```python
from build123d import *

# Parameters (mm, degrees)
BOSS_EXTRUDE3_DEPTH = 4.5
CIRPATTERN1_COUNT   = 12
CIRPATTERN2_COUNT   = 6
SKETCH11_R          = 6.35
CUT_EXTRUDE1_DEPTH  = 10


with BuildPart() as part:
    # Sketch5 → Boss-Extrude3 (new body)
    with BuildSketch(Plane(origin=(0, 0, 0), x_dir=(1, 0, 0), z_dir=(0, 1, 0))):
        with BuildLine():
            ThreePointArc((-45.876558414, 184.378256278), (0.010243817, -189.999999724), (45.856676704, 184.383202059))
            ThreePointArc((45.856676704, 184.383202059), (37.985823171, 188.339968607), (32.578557994, 195.294666309))
            ThreePointArc((32.578557994, 195.294666309), (-0.011645544, 215.998911827), (-32.599616361, 195.291152239))
            ThreePointArc((-32.599616361, 195.291152239), (-38.006131584, 188.335871514), (-45.876558414, 184.378256278))
        make_face()
        with BuildLine():
            Line((-47.367120943, -99.136010081), (-47.045154091, -81.484597135))
            Line((-47.045154091, -81.484597135), (-62.170742689, -90.589135081))
            ThreePointArc((-62.170742689, -90.589135081), (-127.630493883, -73.6875), (-109.537863632, -8.546875))
            Line((-109.537863632, -8.546875), (-94.090308181, 0))
            Line((-94.090308181, 0), (-109.537863632, 8.546875))
            ThreePointArc((-109.537863632, 8.546875), (-127.630493883, 73.6875), (-62.170742689, 90.589135081))
            Line((-62.170742689, 90.589135081), (-47.045154091, 81.484597135))
            Line((-47.045154091, 81.484597135), (-47.367120943, 99.136010081))
            ThreePointArc((-47.367120943, 99.136010081), (0, 147.375), (47.367120943, 99.136010081))
            Line((47.367120943, 99.136010081), (47.045154091, 81.484597135))
            Line((47.045154091, 81.484597135), (62.170742689, 90.589135081))
            ThreePointArc((62.170742689, 90.589135081), (127.630493883, 73.6875), (109.537863632, 8.546875))
            Line((109.537863632, 8.546875), (94.090308181, 0))
            Line((94.090308181, 0), (109.537863632, -8.546875))
            ThreePointArc((109.537863632, -8.546875), (127.630493883, -73.6875), (62.170742689, -90.589135081))
            Line((62.170742689, -90.589135081), (47.045154091, -81.484597135))
            Line((47.045154091, -81.484597135), (47.367120943, -99.136010081))
            ThreePointArc((47.367120943, -99.136010081), (0, -147.375), (-47.367120943, -99.136010081))
        make_face(mode=Mode.SUBTRACT)
    extrude(amount=-BOSS_EXTRUDE3_DEPTH)

    # Sketch7 → CSK for M5 Flat Head Machine Screw1 (revolve, cut)
    with BuildSketch(Plane(origin=(-170, 0, 0), x_dir=(0, 0, 1), z_dir=(1, 0, 0))):
        Polygon((0, 0), (0, 4.5), (2.75, 4.5), (2.75, 2.45), (5.2, 0), align=None)
    csk_for_m5_flat_head_machine_screw1 = revolve(axis=Axis((-170, 6.35, 0), (0, -1, 0)), mode=Mode.SUBTRACT)

    # CirPattern1: CSK for M5 Flat Head Machine Screw1 ×12 about axis, 1 skipped
    cirpattern1_axis = Axis((0, 0, 0), (0, 1, 0))
    add([csk_for_m5_flat_head_machine_screw1.rotate(cirpattern1_axis, i * 360 / CIRPATTERN1_COUNT) for i in range(1, CIRPATTERN1_COUNT) if i not in (9,)], mode=Mode.SUBTRACT)

    # Sketch9 → CSK for M5 Flat Head Machine Screw2 (revolve, cut)
    with BuildSketch(Plane(origin=(-140, 0, 0), x_dir=(0, 0, 1), z_dir=(1, 0, 0))):
        Polygon((0, 0), (0, 4.5), (2.75, 4.5), (2.75, 2.45), (5.2, 0), align=None)
    csk_for_m5_flat_head_machine_screw2 = revolve(axis=Axis((-140, 6.35, 0), (0, -1, 0)), mode=Mode.SUBTRACT)

    # CirPattern2: CSK for M5 Flat Head Machine Screw2 ×6 about axis
    cirpattern2_axis = Axis((0, 0, 0), (0, 1, 0))
    for i in range(1, CIRPATTERN2_COUNT):
        add(csk_for_m5_flat_head_machine_screw2.rotate(cirpattern2_axis, i * 360 / CIRPATTERN2_COUNT), mode=Mode.SUBTRACT)

    # Sketch11 → Cut-Extrude1 (cut)
    with BuildSketch(Plane(origin=(0, 0, 0), x_dir=(1, 0, 0), z_dir=(0, 1, 0))):
        with Locations((-0.009704669, 179.999999411)):
            Circle(SKETCH11_R)
    extrude(amount=-CUT_EXTRUDE1_DEPTH, mode=Mode.SUBTRACT)


solid = part.part
```
Can you work these out from the model? Positions are in its coordinate system, mm. A direction names the side the tool comes from. Coordinates: 2 decimals unless noted, no trailing zeros. Loops run counter-clockwise (first coordinate to the right, second up) from the corner with the lowest first, then second, coordinate; pieces in that order, holes last. Notation, with made-up numbers: M -11.5,-27 L 36.5,-27 A23 ccw 36.5,10 Z; hole C 64.25,-24 d4. An arc over 180 degrees is marked long. Put each result on its own line as item: value. Start each with the question number.
(1) Which directions (+Z, -Z, +X, -X, +Y, -Y) give clear straight access to the entire face, cutting with the end or side of a thin tool? Please do faces 4 (the face through (-147.85, -2.3, -87.83)), 5 (the face through (54.71, -2.22, 86.1)).
(2) Imagine slicing it at A-A on z = -136. List the corners of the cut face in (x, y) for me, and give its area (3 significant figures).
(3) I need wall thicknesses on probe 1 along X at (y, z) = (-2.95, 0); probe 2 along Z at (x, y) = (127.5, -1.15); probe 3 along X at (y, z) = (-1.15, 1). Which ranges of each line are inside material? Lowest first, please.
(4) Will these pins go through, and if not, where does the flat tip stop? pin 1 Ø3.5 at (x, z) = (-147.22, -85) entering from +Y; pin 2 Ø2 at (y, z) = (-0.5, -133) entering from -X; pin 3 Ø6.5 at (x, z) = (-70, 121.24) entering from +Y; pin 4 Ø7 at (x, z) = (-70, -121.24) entering from +Y.
(5) Imagine slicing it at C-C on x = 102.5. List the corners of the cut face in (y, z) for me, and give its area (3 significant figures).
(6) We'd pull the mould along X, two halves only. Please class faces 1 (the face through (69.87, -2.3, -124.14)), 2 (the face through (0.559, -2.218, -215.994)), 3 (the face through (-45, 0, 119)): +X half, -X half, draft (parallel to the pull), parting line (faces both ways), or undercut.
(7) Imagine slicing it at B-B on x = -39. List the corners of the cut face in (y, z) for me, and give its area (3 significant figures).
Worked answers:
1. face 4: +Y
1. face 5: +Y, -Y
2. outline: M -132.68,-4.5 L -30.8,-4.5 L -30.8,0 L -132.68,0 Z; M 30.8,-4.5 L 132.68,-4.5 L 132.68,0 L 30.8,0 Z
2. area: 917 mm2
3. probe 1: x = -190 to -172.75, -167.25 to -142.75, -137.25 to -94.09, 94.09 to 137.25, 142.75 to 167.25, 172.75 to 190
3. probe 2: z = -140.87 to -73.91, -26.09 to 26.09, 73.91 to 140.87
3. probe 3: x = -190 to -173.92, -166.08 to -143.92, -136.08 to -95.9, 95.9 to 136.08, 143.92 to 166.08, 173.92 to 190
4. pin 1: passes through
4. pin 2: stops at x = -136.66
4. pin 3: stops at y = -1.95
4. pin 4: stops at y = -1.7
5. outline: M -4.5,-159.98 L 0,-159.98 L 0,-94.63 L -4.5,-94.63 Z; M -4.5,-4.65 L 0,-4.65 L 0,4.65 L -4.5,4.65 Z; M -4.5,94.63 L 0,94.63 L 0,159.98 L -4.5,159.98 Z
5. area: 630 mm2
6. face 1: undercut
6. face 2: parting line
6. face 3: draft
7. outline: M -4.5,-187.57 L 0,-187.57 L 0,-126.9 L -4.5,-126.9 Z; M -4.5,126.9 L 0,126.9 L 0,185.95 L -4.5,185.95 Z
7. area: 539 mm2
